Autodesk Inventor part; units mm, degrees
ref_plane "YZ Plane" through (0, 0, 0) normal (1, 0, 0) x (0, 1, 0)
ref_plane "XZ Plane" through (0, 0, 0) normal (0, 1, 0) x (-1, 0, 0)
ref_plane "XY Plane" through (0, 0, 0) normal (0, 0, 1) x (1, 0, 0)
sketch "Sketch1" plane through (0, 0, 0) normal (0, 0, 1) x (1, 0, 0)
  line L0 (0, 0) -> (0, 14.2875)
  line L1 (0, 14.2875) -> (9.8425, 14.2875) construction
  line L2 (9.8425, 14.2875) -> (14.605, 14.2875)
  line L3 (14.605, 14.2875) -> (14.605, 0)
  line L4 (14.605, 0) -> (11.43, 1.5875)
  line L5 (11.43, 1.5875) -> (9.8425, 14.2875)
  dimension "d1" = 19.685
  dimension "d2" = 1.5875
  dimension "d3" = 3.175
  dimension "d5" = 14.2875
  dimension "d6" = 12.7
revolve "Revolution1" add sketch "Sketch1" angle 360 about axis through (0, 0, 0) along (0, 1, 0)
sketch "Sketch2" plane through (0, 14.2875, 0) normal (0, 1, 0) x (1, 0, 0)
  line L0 (17.78, -26.9875) -> (-17.78, -26.9875)
  line L1 (-17.78, -26.9875) -> (-17.78, 26.9875)
  line L2 (-17.78, 26.9875) -> (17.78, 26.9875)
  line L3 (17.78, 26.9875) -> (17.78, -26.9875)
  line L4 (17.78, -26.9875) -> (-17.78, 26.9875) construction
  line L5 (-17.78, -26.9875) -> (17.78, 26.9875) construction
  circle A0 centre (0, 0) radius 14.605
  point P0 (0, -14.605)
  point P1 (-14.605, 0)
  dimension "d9" = 3.175
  dimension "d22" = 53.975
extrude "Extrusion1" add sketch "Sketch2" against normal blind 1.5875
sketch "Sketch3" plane through (-17.78, 14.2875, -26.9875) normal (0, 1, 0) x (1, 0, 0)
  line L0 (17.78, -46.0375) -> (17.78, -7.9375) construction
  line L1 (5.08, -49.2125) -> (30.48, -49.2125)
  line L2 (30.48, -49.2125) -> (30.48, -4.7625)
  line L3 (30.48, -4.7625) -> (5.08, -4.7625)
  line L4 (5.08, -4.7625) -> (5.08, -49.2125)
  line L5 (5.08, -49.2125) -> (30.48, -4.7625) construction
  line L6 (30.48, -49.2125) -> (5.08, -4.7625) construction
  point P0 (17.78, -26.9875)
  point P1 (17.78, -26.9875)
  dimension "d12" = 38.1
  dimension "d20" = 44.45
  dimension "d21" = 25.4
hole "Hole1" at (12.7, 14.2875, 22.225) at (12.7, 14.2875, -22.225) at (-12.7, 14.2875, -22.225) at (-12.7, 14.2875, 22.225) at (0, 14.2875, -19.05) at (0, 14.2875, 19.05) direction (0, -1, 0) diameter 5.1054 end through all
sketch "Sketch4" plane through (0, 12.7, 0) normal (0, -1, 0) x (1, 0, 0)
  circle A0 centre (0, 19.05) radius 2.5527
  circle A1 centre (0, 19.05) radius 5.08
  circle A2 centre (0, -19.05) radius 2.5527
  circle A3 centre (0, -19.05) radius 5.08
  point P0 (0, 0)
  dimension "d23" = 10.16
extrude "Extrusion2" cut sketch "Sketch4" along normal up to surface
properties part number "Gripper_3DPrint"
Work out the finished part from the listing and answer in its coordinate system (mm). A direction names the side the tool comes from. Round coordinates to 2 decimals unless told otherwise and drop trailing zeros. Order: outer loops, then holes, each group sorted by start corner. A loop starts at its lowest first (then second) coordinate and runs counter-clockwise, first axis right, second up. Notation, with made-up numbers: M -28.75,31 L -6.75,31 A21 ccw -6.75,55 Z; hole C 79,64 d1. An arc over 180 degrees is marked long. One line per item, written item: value.
Q1. For faces 4 (the face through (0.03, 6.44, 13.97)), 5 (the face through (-14.6, 6.3, 0.3)), 6 (the face through (-8.2, 12.7, -12.4)), determine the directions among +Z, -Z, +X, -X, +Y, -Y from which every point of the face is accessible in a straight line to the end or side of a thin tool.
Derived:
face 4: +Z, -Y
face 5: -X, -Y
face 6: -Y
Q2. Flat-ended cylindrical pins translate along their axes: pin 1 (4 mm diameter, centred on x = 3.5, y = 9.5, fed in from +Z); pin 2 (2 mm diameter, centred on y = 3, z = -12.5, fed in from +X); pin 3 (2 mm diameter, centred on x = -7.5, y = 11, fed in from -Z). Find the tip coordinate at first contact, or state that the pin passes through.
Derived:
pin 1: z = 14.45
pin 2: x = 9
pin 3: z = -13.08
Q3. Find section D-D on x = -12.7. Give the number of separate pieces and of enclosed holes in the cut face, then the cut area to 3 significant figures.
Derived:
separate pieces: 3
enclosed holes: 0
area: 244 mm²
Q4. Find section A-A on z = 19.05. Write down the section's boundary in (x, y).
Derived:
outline: M -17.78,12.7 L -2.55,12.7 L -2.55,14.29 L -17.78,14.29 Z; M 2.55,12.7 L 17.78,12.7 L 17.78,14.29 L 2.55,14.29 Z
Q5. Find section B-B on x = 0. Write down the section's boundary in (y, z).
Derived:
outline: M 0.32,-13.97 L 12.7,-13.97 L 12.7,-16.5 L 14.29,-16.5 L 14.29,-9.84 L 1.59,-11.43 Z; M 0.32,13.97 L 1.59,11.43 L 14.29,9.84 L 14.29,16.5 L 12.7,16.5 L 12.7,13.97 Z; M 12.7,-26.99 L 14.29,-26.99 L 14.29,-21.6 L 12.7,-21.6 Z; M 12.7,21.6 L 14.29,21.6 L 14.29,26.99 L 12.7,26.99 Z
Q6. Find section C-C on y = 8.75. Write down the section's boundary in (x, z) (3 decimals), then the cut area to 3 significant figures.
Derived:
outline: M -2.148,-14.446 A5.08 cw 2.148,-14.446 A14.605 ccw 2.148,14.446 A5.08 cw -2.148,14.446 A14.605 ccw Z; hole C 0,0 d21.069
area: 318 mm²
Q7. Determine the mould class of faces 1 (the face through (-12.812, 13.483, 19.675)), 2 (the face through (-8, 14.288, -6)), 3 (the face through (0, 14, -26.988)) for opening direction Z: released by +Z, released by -Z, zero draft, split by the parting line, or undercut.
Derived:
face 1: undercut
face 2: zero draft
face 3: released by -Z
Q8. Straight lines are drawn through the part: line 1 (Z direction, x = -12.7, y = 13.5); line 2 (X direction, y = 13.6, z = -19.05); line 3 (Z direction, x = 0, y = 13.25). For each, find the intervals that lie inside material, in ascending order.
Derived:
line 1: -26.99 to -24.78, -19.67 to 19.67, 24.78 to 26.99
line 2: -17.78 to -2.55, 2.55 to 17.78
line 3: -26.99 to -21.6, -16.5 to -9.97, 9.97 to 16.5, 21.6 to 26.99
